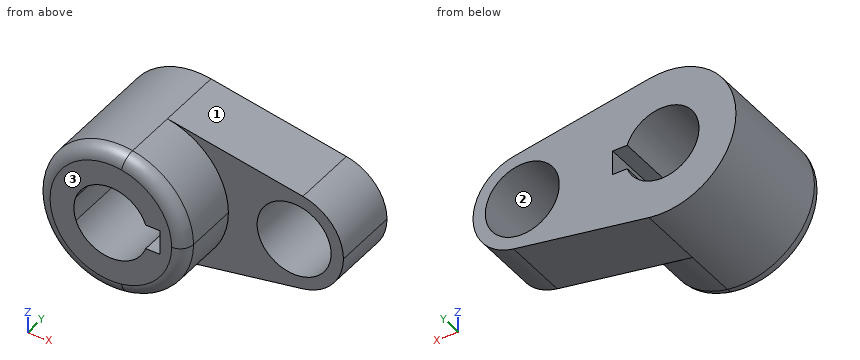
from build123d import *

# Parameters (mm, degrees)
F0_R     = 14.2875
F1_DEPTH = 25.4
F2_DEPTH = 50.8
F3_R     = 5.08


with BuildPart() as f1:
    # F0 (on Front) → F1 (new body)
    with BuildSketch(Plane.XZ):
        with BuildLine():
            ThreePointArc((5.042647, -28.126541), (21.916025, -18.336262), (28.575, 0))
            ThreePointArc((28.575, 0), (21.916025, 18.336262), (5.042647, 28.126541))
            ThreePointArc((5.042647, 28.126541), (-28.575, 0), (5.042647, -28.126541))
        make_face()
        with BuildLine():
            ThreePointArc((-13.470384, 4.7625), (0, 14.2875), (13.470384, 4.7625))
            Line((13.470384, 4.7625), (19.05, 4.7625))
            Line((19.05, 4.7625), (19.05, -4.7625))
            Line((19.05, -4.7625), (13.470384, -4.7625))
            ThreePointArc((13.470384, -4.7625), (0, -14.2875), (-13.470384, -4.7625))
            Line((-13.470384, -4.7625), (-19.05, -4.7625))
            Line((-19.05, -4.7625), (-19.05, 4.7625))
            Line((-19.05, 4.7625), (-13.470384, 4.7625))
        make_face(mode=Mode.SUBTRACT)
        with BuildLine():
            ThreePointArc((-13.470384, -4.7625), (-14.2875, 0), (-13.470384, 4.7625))
            Line((-13.470384, 4.7625), (-19.05, 4.7625))
            Line((-19.05, 4.7625), (-19.05, -4.7625))
            Line((-19.05, -4.7625), (-13.470384, -4.7625))
        make_face()
        with BuildLine():
            ThreePointArc((5.042647, 28.126541), (21.916025, 18.336262), (28.575, 0))
            ThreePointArc((28.575, 0), (21.916025, -18.336262), (5.042647, -28.126541))
            Line((5.042647, -28.126541), (57.336765, -18.751028))
            ThreePointArc((57.336765, -18.751028), (34.925, 0), (57.336765, 18.751028))
            Line((57.336765, 18.751028), (5.042647, 28.126541))
        make_face()
        with BuildLine():
            ThreePointArc((73.025, 0), (68.585683, 12.224174), (57.336765, 18.751028))
            ThreePointArc((57.336765, 18.751028), (34.925, 0), (57.336765, -18.751028))
            ThreePointArc((57.336765, -18.751028), (68.585683, -12.224174), (73.025, 0))
        make_face()
        with Locations((53.975, 0)):
            Circle(F0_R, mode=Mode.SUBTRACT)
    extrude(amount=F1_DEPTH)

    # F0 (on Front) → F2 (join)
    with BuildSketch(Plane.XZ):
        with BuildLine():
            ThreePointArc((5.042647, -28.126541), (21.916025, -18.336262), (28.575, 0))
            ThreePointArc((28.575, 0), (21.916025, 18.336262), (5.042647, 28.126541))
            ThreePointArc((5.042647, 28.126541), (-28.575, 0), (5.042647, -28.126541))
        make_face()
        with BuildLine():
            ThreePointArc((-13.470384, 4.7625), (0, 14.2875), (13.470384, 4.7625))
            Line((13.470384, 4.7625), (19.05, 4.7625))
            Line((19.05, 4.7625), (19.05, -4.7625))
            Line((19.05, -4.7625), (13.470384, -4.7625))
            ThreePointArc((13.470384, -4.7625), (0, -14.2875), (-13.470384, -4.7625))
            Line((-13.470384, -4.7625), (-19.05, -4.7625))
            Line((-19.05, -4.7625), (-19.05, 4.7625))
            Line((-19.05, 4.7625), (-13.470384, 4.7625))
        make_face(mode=Mode.SUBTRACT)
        with BuildLine():
            ThreePointArc((-13.470384, -4.7625), (-14.2875, 0), (-13.470384, 4.7625))
            Line((-13.470384, 4.7625), (-19.05, 4.7625))
            Line((-19.05, 4.7625), (-19.05, -4.7625))
            Line((-19.05, -4.7625), (-13.470384, -4.7625))
        make_face()
    extrude(amount=F2_DEPTH)

    # F3
    f3_edges = [f1.edges().sort_by_distance(p)[0] for p in [
        (-5.042647, -50.8, 28.126541),
    ]]
    fillet(f3_edges, radius=F3_R)


solid = f1.part
Design review of the part built by this model. Coordinates are the model's own, in mm. Face numbers are marked on the shaded views. Round coordinates to 2 decimals unless told otherwise and drop trailing zeros. Order: outer loops, then holes, each group sorted by start corner. A loop starts at its lowest first (then second) coordinate and runs counter-clockwise, first axis right, second up. Notation, with made-up numbers: M -35,-31 L -13,-31 A9 cw -13,-15 Z; hole C 10.5,51 d8. An arc over 180 degrees is marked long. Answer as CSV lines item,"result". Start each with the question number.
1) The part is to be moulded in two halves that separate along X. For the marked faces 1, 2 and 3, say which applies: +X half, -X half, draft (parallel to the pull), parting line (faces both ways), or undercut.
2) Add section B-B (x = 54). Give the boundary of the cut face in (y, z), then the cut area to 3 significant figures.
3) For pin 1 Ø10 at (y, z) = (-34, -19) entering from +X; pin 2 Ø6 at (x, y) = (17.5, -35) entering from -Z; pin 3 Ø1 at (y, z) = (-37, 16.5) entering from +X; pin 4 Ø17 at (x, z) = (53.975, 0) entering from +Y, all flat-tipped, find the tip position at first contact; note any pin that passes through.
4) Add section A-A (y = -3). Give the number of separate pieces and of enclosed holes in the cut face, then the cut area to 3 significant figures.
5) Wall thickness on line 1 along X through (y, z) = (-6, -2); line 2 along X through (y, z) = (-2.5, 13); line 3 along X through (y, z) = (-33, -9): over which ranges is each line inside the solid? List them lowest first. Write a range as [from, to].
Resolved:
1,face 1,"+X half"
1,face 2,"undercut"
1,face 3,"draft"
2,outline,"M -25.4,-19.35 L 0,-19.35 L 0,-14.29 L -25.4,-14.29 Z; M -25.4,14.29 L 0,14.29 L 0,19.35 L -25.4,19.35 Z"
2,area,"257 mm^2"
3,pin 1,"x = 24.91"
3,pin 2,"z = -24.62"
3,pin 3,"x = 23.68"
3,pin 4,"through"
4,separate pieces,"1"
4,enclosed holes,"2"
4,area,"3,130 mm^2"
5,line 1,"[-28.5, -14.15], [19.05, 39.83], [68.12, 72.92]"
5,line 2,"[-25.45, -5.93], [5.93, 48.05], [59.9, 67.9]"
5,line 3,"[-27.12, -11.1], [11.1, 27.12]"
